from build123d import *

# Parameters (mm, degrees)
F0_R      = 18.415
F1_DEPTH  = 22.098
F2_R      = 5.969
F2_R_2    = 3.048
F3_DEPTH  = 6.5
F4_DEPTH  = 15.494
F5_R      = 17.399
F6_DEPTH  = 30.734
F7_R      = 16.891
F8_DEPTH  = 15.494
F9_R      = 2.1209
F9_R_2    = 2.11499958
F10_DEPTH = 11.176


with BuildPart() as f1:
    # F0 (on Front) → F1 (new body)
    with BuildSketch(Plane.XZ):
        Circle(F0_R)
    extrude(amount=F1_DEPTH)

    # F2 (on face) → F3 (join)
    with BuildSketch(Plane(origin=(0, 0, 0), x_dir=(-1, 0, 0), z_dir=(0, 1, 0))):
        with Locations((0, -8.4149946)):
            Circle(F2_R)
        with Locations((0, -8.4149946)):
            Circle(F2_R_2, mode=Mode.SUBTRACT)
    extrude(amount=F3_DEPTH)

    # F4 (add): a face of the model
    f4_faces = [f1.faces().sort_by_distance(p)[0] for p in [
        (0, 0, -8.4149946),
    ]]
    extrude(f4_faces, amount=F4_DEPTH)

    # F5 (on face) → F6 (join)
    with BuildSketch(Plane.XZ.offset(22.098)):
        Circle(F5_R)
    extrude(amount=F6_DEPTH)

    # F7 (on face) → F8 (join)
    with BuildSketch(Plane.XZ.offset(52.832)):
        Circle(F7_R)
    extrude(amount=F8_DEPTH)

    # F9 (on face) → F10 (cut)
    with BuildSketch(Plane(origin=(0, 0, 0), x_dir=(-1, 0, 0), z_dir=(0, 1, 0))):
        with Locations((-11.2272249535, -10.0982319564)):
            Circle(F9_R)
        with Locations((0, 15.875)):
            Circle(F9_R_2)
        with Locations((11.2272249535, -10.0982319564)):
            Circle(F9_R)
    extrude(amount=-F10_DEPTH, mode=Mode.SUBTRACT)


solid = f1.part
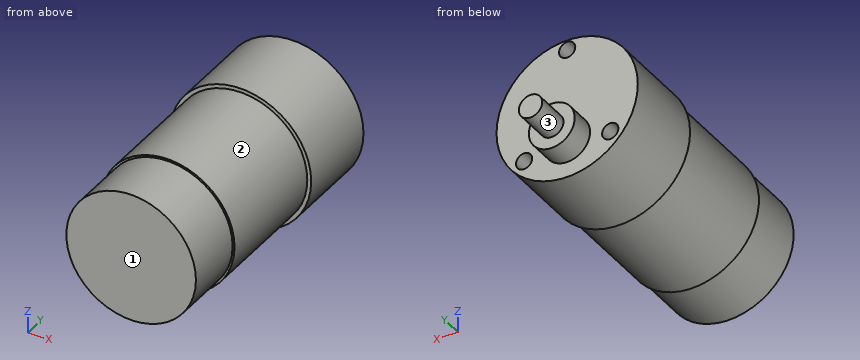
Model file for the job. Use its own axes, mm. Face numbers are marked on the shaded views. A direction names the side the tool comes from. Give positions to 0.01 mm unless a question says otherwise; leave off trailing zeros. Loops run counter-clockwise (first coordinate to the right, second up) from the corner with the lowest first, then second, coordinate; pieces in that order, holes last.
Item 1: Slice it at B-B (x = 0). Write the cut outline in (y, z) (3 decimals), plus the area to 3 significant figures.
Check values:
outline: (-68.326, -16.891) - (-52.832, -16.891) - (-52.832, -17.399) - (-22.098, -17.399) - (-22.098, -18.415) - (0, -18.415) - (0, -14.384) - (6.5, -14.384) - (6.5, -11.463) - (15.494, -11.463) - (15.494, -5.367) - (6.5, -5.367) - (6.5, -2.446) - (0, -2.446) - (0, 13.76) - (-11.176, 13.76) - (-11.176, 17.99) - (0, 17.99) - (0, 18.415) - (-22.098, 18.415) - (-22.098, 17.399) - (-52.832, 17.399) - (-52.832, 16.891) - (-68.326, 16.891) - close
area: 2,490 mm2
Item 2: Slice it at C-C (y = -20.5). Write the cut outline in (x, z) (3 decimals).
Check values:
outline: circle Ø36.83 at (0, 0)
Item 3: Slice it at A-A (z = 0). Write the cut outline in (x, y) (3 decimals).
Check values:
outline: (-18.415, -22.098) - (-17.399, -22.098) - (-17.399, -52.832) - (-16.891, -52.832) - (-16.891, -68.326) - (16.891, -68.326) - (16.891, -52.832) - (17.399, -52.832) - (17.399, -22.098) - (18.415, -22.098) - (18.415, 0) - (-18.415, 0) - close
Item 4: Drill centre lines: line 1 along Z through (x, y) = (0, -4.5) (3 decimals); line 2 along Y through (x, z) = (-8, 7.5); line 3 along Z through (x, y) = (-15, -40). Where is each one in solid material? Low to high.
Check values:
line 1: z = -18.415 to 13.76, 17.99 to 18.415
line 2: y = -68.33 to 0
line 3: z = -8.82 to 8.82
Item 5: Slice it at D-D (z = 9). Write the cut outline in (x, y), plus the area to 3 significant figures.
Check values:
outline: (-16.07, -22.1) - (-14.89, -22.1) - (-14.89, -52.83) - (-14.29, -52.83) - (-14.29, -68.33) - (14.29, -68.33) - (14.29, -52.83) - (14.89, -52.83) - (14.89, -22.1) - (16.07, -22.1) - (16.07, 0) - (-16.07, 0) - close
area: 2,070 mm2
Item 6: Which spindle directions (+Z, -Z, +X, -X, +Y, -Y) get a long thin tool onto all of the face, cutting with end or side? Do the marked faces 1, 2 and 3. Say none if no direction does.
Check values:
face 1: +Z, -Z, +X, -X, -Y
face 2: -Y
face 3: +Y
Item 7: Drop flat-ended pins along their axis: P1, Ø2, axis at x = -3, y = 0, coming from the -Z side; P2, Ø7, axis at x = 11.23, z = -10.1, coming from the +Y side; P3, Ø4, axis at x = 1, y = -31.5, coming from the +Z side. Give the stop position or say it passes through.
Check values:
P1: stops at z = -18.31
P2: stops at y = 0
P3: stops at z = 17.4
